Could you check a few things on this model? Use its own coordinates, in mm. Give positions to 0.01 mm unless a question says otherwise; leave off trailing zeros. Order: outer loops, then holes, each group sorted by start corner. A loop starts at its lowest first (then second) coordinate and runs counter-clockwise, first axis right, second up.
(1) Imagine slicing it at D-D, the plane z = 3.25. Write out the boundary of the cut face in (x, y), then the cut area to 3 significant figures.
(2) Will these pins go through, and if not, where does the flat tip stop? pin 1 (12 mm diameter, centred on x = 0, z = 5, fed in from -Y); pin 2 (12 mm diameter, centred on y = -12, z = -9, fed in from +X); pin 3 (5 mm diameter, centred on x = 18.5, z = -3.5, fed in from -Y).
(3) Imagine slicing it at A-A, the plane y = 0. Write out the boundary of the cut face in (x, z).
(4) Imagine slicing it at C-C, the plane x = 8. Write out the boundary of the cut face in (y, z).
(5) If we mould it in two halves opening along X, with no side actions, what happens to faces 1 (the flat face through (18, -6, -12.5)), 2 (the cylindrical face through (-5.961, -26.846, 0.175)), 3 (the cylindrical face through (-1.1, -25.6, 0.2))? For each: released by +X, released by -X, zero draft, split by the parting line, or undercut.
(6) If I drill on probe 1 along Y at (x, z) = (0, -1.75); probe 2 along Y at (x, z) = (19.5, -5.5); probe 3 along Y at (x, z) = (11.5, 5.75), over which ranges is the centre line in solid material (lowest first)?
(7) Imagine slicing it at B-B, the plane x = 0. Write out the boundary of the cut face in (y, z).
from build123d import *

# Parameters (mm, degrees)
SKETCH2_R                       = 27.5
SKETCH2_R_2                     = 18
BOSS_EXTRUDE1_DEPTH             = 12.5
TAP_DRILL_FOR_M5X0_8_TAP1_D     = 4.2
TAP_DRILL_FOR_M5X0_8_TAP1_DEPTH = 25.001
CIRPATTERN5_COUNT               = 6


with BuildPart() as part:
    # Sketch2 → Boss-Extrude1 (new body, symmetric)
    with BuildSketch(Plane.XY):
        Circle(SKETCH2_R)
        Circle(SKETCH2_R_2, mode=Mode.SUBTRACT)
    extrude(amount=BOSS_EXTRUDE1_DEPTH, both=True)

    # Tap Drill for M5x0.8 Tap1
    with Locations(Plane(origin=(0, 0, -12.5), x_dir=(-1, 0, 0), z_dir=(0, 0, -1))):
        with Locations((0, 23.8125)):
            tap_drill_for_m5x0_8_tap1 = Hole(TAP_DRILL_FOR_M5X0_8_TAP1_D / 2, depth=TAP_DRILL_FOR_M5X0_8_TAP1_DEPTH)

    # CirPattern5: Tap Drill for M5x0.8 Tap1 ×6 about axis
    cirpattern5_axis = Axis((0, 0, 0), (0, 0, 1))
    for i in range(1, CIRPATTERN5_COUNT):
        add(tap_drill_for_m5x0_8_tap1.rotate(cirpattern5_axis, i * 360 / CIRPATTERN5_COUNT), mode=Mode.SUBTRACT)


solid = part.part
Answer block:
1. outline: circle Ø55 at (0, 0); hole circle Ø4.2 at (-20.62, -11.91); hole circle Ø4.2 at (-20.62, 11.91); hole circle Ø36 at (0, 0); hole circle Ø4.2 at (0, -23.81); hole circle Ø4.2 at (0, 23.81); hole circle Ø4.2 at (20.62, -11.91); hole circle Ø4.2 at (20.62, 11.91)
1. area: 1,270 mm2
2. pin 1: stops at y = -27.5
2. pin 2: stops at x = 26.84
2. pin 3: stops at y = -22.37
3. outline: (-27.5, -12.5) - (-18, -12.5) - (-18, 12.5) - (-27.5, 12.5) - close; (18, -12.5) - (27.5, -12.5) - (27.5, 12.5) - (18, 12.5) - close
4. outline: (-26.31, -12.5) - (-16.12, -12.5) - (-16.12, 12.5) - (-26.31, 12.5) - close; (16.12, -12.5) - (26.31, -12.5) - (26.31, 12.5) - (16.12, 12.5) - close
5. face 1: zero draft
5. face 2: split by the parting line
5. face 3: undercut
6. probe 1: y = -27.5 to -25.91, -21.71 to -18, 18 to 21.71, 25.91 to 27.5
6. probe 2: y = -19.39 to -13.68, -10.13 to 10.13, 13.68 to 19.39
6. probe 3: y = -24.98 to -13.85, 13.85 to 24.98
7. outline: (-27.5, -12.5) - (-25.91, -12.5) - (-25.91, 12.5) - (-27.5, 12.5) - close; (-21.71, -12.5) - (-18, -12.5) - (-18, 12.5) - (-21.71, 12.5) - close; (18, -12.5) - (21.71, -12.5) - (21.71, 12.5) - (18, 12.5) - close; (25.91, -12.5) - (27.5, -12.5) - (27.5, 12.5) - (25.91, 12.5) - close
